Source: CAD feature listing. Evaluate the final solid. Frame: model axes, mm. Give positions to 0.01 mm unless a question says otherwise; leave off trailing zeros. Loops run counter-clockwise (first coordinate to the right, second up) from the corner with the lowest first, then second, coordinate; pieces in that order, holes last. Notation, with made-up numbers: (44.25, 14) -> (84.25, 14) arc R19 ccw to (84.25, 41) -> close; hole circle Ø3 at (11, 89.5). An arc over 180 degrees is marked (long way). Answer as a JSON object with one key per item and string values. Group by question number.
Autodesk Inventor part; units mm, degrees
ref_plane "YZ Plane" through (0, 0, 0) normal (1, 0, 0) x (0, 1, 0)
ref_plane "XZ Plane" through (0, 0, 0) normal (0, 1, 0) x (-1, 0, 0)
ref_plane "XY Plane" through (0, 0, 0) normal (0, 0, 1) x (1, 0, 0)
sketch "スケッチ1" plane through (0, 0, 0) normal (0, 0, 1) x (1, 0, 0)
  circle A0 centre (0, 0) radius 2
  circle A1 centre (0, 0) radius 4
  dimension "d0" = 4
  dimension "d1" = 8
extrude "押し出し1" add sketch "スケッチ1" along normal mid plane 182 contours A0 | A1
sketch "スケッチ3" plane through (0, 0, 91) normal (0, 0, 1) x (1, 0, 0)
  circle A0 centre (0, 0) radius 2
  dimension "d5" = 4
extrude "押し出し2" cut sketch "スケッチ3" against normal blind 10
sketch "スケッチ4" plane through (0, 0, -91) normal (0, 0, -1) x (-1, 0, 0)
  circle A0 centre (0, 0) radius 2
  dimension "d8" = 4
extrude "押し出し3" cut sketch "スケッチ4" against normal blind 10
properties part number "シャフト182mm" material "アルミニウム 7075"
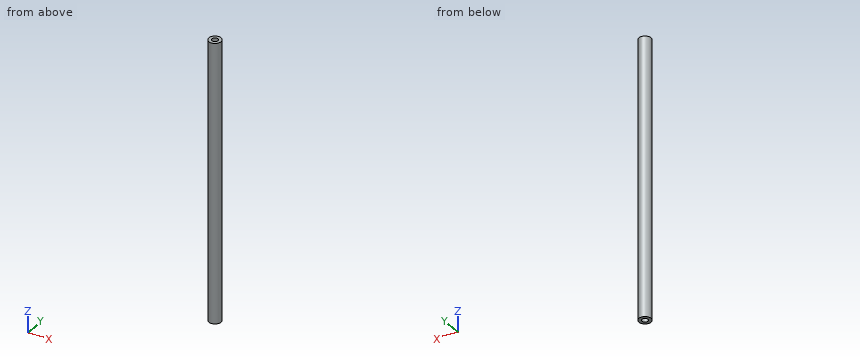
(1) Section query A-A on x = 0. Return the cut outline in (y, z), plus the area to 3 significant figures.
(2) Section query B-B on z = -69. Return the cut outline in (x, y), plus the area to 3 significant figures.
(3) First-contact query: pin 1 (4.5 mm diameter, centred on x = 0, y = 0, fed in from +Z); pin 2 (2 mm diameter, centred on x = 2, z = 31, fed in from -Y); pin 3 (2.5 mm diameter, centred on x = 0, y = 0, fed in from +Z); pin 4 (3 mm diameter, centred on y = 2, z = 54.5, fed in from -X). Flat tips, straight axial feed; report the tip coordinate or a pass-through.
(4) Material intervals for line 1 (Y direction, x = 0, z = 87.75); line 2 (Y direction, x = 0.5, z = -44), sorted ascending. Write a range as from..to.
Result:
{
 "1": {"outline": "(-4, -91) -> (-2, -91) -> (-2, -81) -> (2, -81) -> (2, -91) -> (4, -91) -> (4, 91) -> (2, 91) -> (2, 81) -> (-2, 81) -> (-2, 91) -> (-4, 91) -> close", "area": "1,380 mm²"},
 "2": {"outline": "circle Ø8 at (0, 0)", "area": "50.3 mm²"},
 "3": {"pin 1": "z = 91", "pin 2": "y = -3.87", "pin 3": "z = 81", "pin 4": "x = -3.97"},
 "4": {"line 1": "-4..-2, 2..4", "line 2": "-3.97..3.97"}
}
